Design review of the part built by this model. Coordinates are the model's own, in mm. A direction names the side the tool comes from. Coordinates: 2 decimals unless noted, no trailing zeros. Use one line per item in the form item = value. Start each with the question number.
(1) The part is to be moulded in two halves that separate along X. For faces 4 (the face through (-169.1, -180, -0.5)), 5 (the face through (81.85, -55.69, 0.01)), 6 (the face through (-66.31, -85.98, 0.01)), 7 (the face through (-31, -25, 3)), say which applies: pulls with the +X half, pulls with the -X half, needs draft (parallel to the pull), parting line crosses it, or undercut.
(2) Clearance check with a flat-ended pin moving along its axis: pin 1 Ø2 at (y, z) = (-31, 2.5) entering from -X. State where the tip first meets the part, or that it passes through.
(3) Tool access review of faces 1 (the face through (-87.03, -68.12, -0.49)), 2 (the face through (60.65, -77.9, -0.49)), 3 (the face through (-68.57, -88.16, 2.43)): name each direction out of +Z, -Z, +X, -X, +Y, -Y from which nothing blocks a thin tool from reaching the whole face with its end or side.
(4) For L1, parallel to X at y = -44.5, z = 1.8; L2, parallel to X at y = -36, z = 1.25; L3, parallel to Y at x = -157, z = -0.55, list the stretches that pass through material, from the lowest coordinate up.
```python
from build123d import *

# Parameters (mm, degrees)
PAD_DEPTH = 1
FILLET_R  = 2


with BuildPart() as part:
    # Sketch → Loft section 0
    with BuildSketch(Plane.XY):
        with BuildLine():
            Line((-4.09576, 2.867882), (-130.282576, -177.345568))
            ThreePointArc((-164.635111, -142.209053), (-168.63735, -180.483273), (-130.282576, -177.345568))
            ThreePointArc((-164.635111, -142.209053), (-86.123884, -66.881649), (-38.476503, 30.934289))
            ThreePointArc((38.22531, 31.782432), (-0.442279, 59.997555), (-38.476503, 30.934289))
            ThreePointArc((38.22531, 31.782432), (82.673152, -56.820578), (153.568717, -126.102055))
            ThreePointArc((118.811047, -160.962527), (156.993603, -164.274662), (153.568717, -126.102055))
            Line((4.09576, 2.867882), (118.811047, -160.962527))
            ThreePointArc((4.09576, 2.867882), (0, 5), (-4.09576, 2.867882))
        make_face()
    # Sketch001 → Loft section 1
    with BuildSketch(Plane.XY.offset(3)):
        with BuildLine():
            Line((-4.09576, 2.867882), (-130.282576, -177.345568))
            ThreePointArc((-155.648016, -152.488447), (-157.625766, -179.877279), (-130.282576, -177.345568))
            ThreePointArc((-155.648016, -152.488447), (-79.841331, -71.777908), (-38.476503, 30.934289))
            ThreePointArc((38.22531, 31.782432), (-0.442279, 59.997555), (-38.476503, 30.934289))
            ThreePointArc((38.22531, 31.782432), (82.673152, -56.820578), (153.568717, -126.102055))
            ThreePointArc((129.282887, -152.184683), (156.461518, -153.143294), (153.568717, -126.102055))
            Line((4.09576, 2.867882), (129.282887, -152.184683))
            ThreePointArc((4.09576, 2.867882), (0, 5), (-4.09576, 2.867882))
        make_face()
    loft()

    # Sketch → Pad (new body)
    with BuildSketch(Plane.XY):
        with BuildLine():
            Line((-4.09576, 2.867882), (-130.282576, -177.345568))
            ThreePointArc((-164.635111, -142.209053), (-168.63735, -180.483273), (-130.282576, -177.345568))
            ThreePointArc((-164.635111, -142.209053), (-86.123884, -66.881649), (-38.476503, 30.934289))
            ThreePointArc((38.22531, 31.782432), (-0.442279, 59.997555), (-38.476503, 30.934289))
            ThreePointArc((38.22531, 31.782432), (82.673152, -56.820578), (153.568717, -126.102055))
            ThreePointArc((118.811047, -160.962527), (156.993603, -164.274662), (153.568717, -126.102055))
            Line((4.09576, 2.867882), (118.811047, -160.962527))
            ThreePointArc((4.09576, 2.867882), (0, 5), (-4.09576, 2.867882))
        make_face()
    extrude(amount=-PAD_DEPTH)

    # Fillet
    fillet_edges = [part.edges().sort_by_distance(p)[0] for p in [
        (0, 5, 3),
        (-67.189168, -87.238843, 3),
        (-157.625766, -179.877279, 3),
        (-79.841331, -71.777908, 3),
        (-0.442279, 59.997555, 3),
        (82.673152, -56.820578, 3),
        (156.461518, -153.143294, 3),
        (66.689324, -74.6584, 3),
    ]]
    fillet(fillet_edges, radius=FILLET_R)


solid = part.part
```
Computed values:
q1.face_4 = parting line crosses it
q1.face_5 = pulls with the +X half
q1.face_6 = undercut
q1.face_7 = needs draft
q2.pin_1 = -60.79
q3.face_1 = +Z, -Z, -X, +Y
q3.face_2 = +Z, -Z, -Y
q3.face_3 = +Z, -Y
q4.L1 = -67.04 to -37.47, 40.24 to 73.94
q4.L2 = -63.73 to -31.33, 32.99 to 68.74
q4.L3 = -187.22 to -136.95
